The listing builds one solid part. Answer for the finished solid, in the listing's coordinates (mm). Face numbers are marked on the shaded views. A direction names the side the tool comes from. Coordinates: 2 decimals unless noted, no trailing zeros. Loops run counter-clockwise (first coordinate to the right, second up) from the corner with the lowest first, then second, coordinate; pieces in that order, holes last. Notation, with made-up numbers: M 67,-18.5 L 115,-18.5 A27 ccw 115,16.5 Z; hole C 89,59 d3. An arc over 180 degrees is marked long. Return JSON: item names as keys, results as strings. Group by question number.
1. The mould has two halves that part along X. Classify the marked faces 1, 2 and 3: pulls with the +X half, pulls with the -X half, needs draft (parallel to the pull), parting line crosses it, or undercut.
2. Section D-D (y = 25.5) is taken. Write down the section's boundary in (x, z), then the cut area to 3 significant figures.
3. Which of the six approach directions +Z, -Z, +X, -X, +Y, -Y give full straight-line access (tool end or side, diameter ignored) to the marked faces 4, 5 and 6?
4. Given P1, Ø1.5, axis at x = 61.5, z = 3.5, coming from the -Y side; P2, Ø24, axis at x = 61.5, z = -19, coming from the +Y side; P3, Ø5, axis at y = 55, z = -24, coming from the -X side; P4, Ø20, axis at x = 118.5, z = 8.5, coming from the +Y side, each flat-ended and moving along its own axis, determine where each tip first touches the part or whether it passes through.
5. Straight lines are drawn through the part: L1, parallel to X at y = 23, z = 0; L2, parallel to Z at x = 34, y = 43; L3, parallel to X at y = 43, z = 0. For each, find the intervals that lie inside material, in ascending order. Write a range as from..to.
6. Section A-A (x = 70) is taken. Write down the section's boundary in (y, z).
7. Section C-C (z = 0) is taken. Write down the section's boundary in (x, y), then the cut area to 3 significant figures.
8. Section B-B (y = 47) is taken. Write down the section's boundary in (x, z), then the cut area to 3 significant figures.
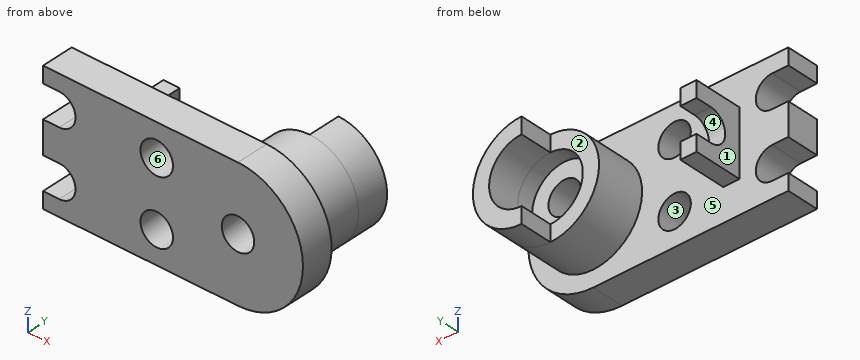
```python
from build123d import *

# Parameters (mm, degrees)
BOSS_EXTRUDE1_DEPTH = 20
CUT_EXTRUDE1_DEPTH  = 20
SKETCH4_R           = 10
CUT_EXTRUDE2_DEPTH  = 20
SKETCH5_R           = 20
BOSS_EXTRUDE2_DEPTH = 20
SKETCH6_R           = 30
BOSS_EXTRUDE3_DEPTH = 30
SKETCH7_R           = 20
CUT_EXTRUDE3_DEPTH  = 10
SKETCH8_R           = 10
CUT_EXTRUDE4_DEPTH  = 72
BOSS_EXTRUDE4_DEPTH = 20
SKETCH10_W          = 10
SKETCH10_H          = 40
BOSS_EXTRUDE5_DEPTH = 30
CUT_EXTRUDE5_DEPTH  = 30


with BuildPart() as part:
    # Sketch2 → Boss-Extrude1 (new body)
    with BuildSketch(Plane(origin=(0, 0, 0), x_dir=(1, 0, 0), z_dir=(0, 1, 0))):
        with BuildLine():
            Line((0, 40), (0, -40))
            Line((0, -40), (120, -40))
            ThreePointArc((120, -40), (160, 0), (120, 40))
            Line((120, 40), (0, 40))
        make_face()
    extrude(amount=BOSS_EXTRUDE1_DEPTH)

    # Sketch3 → Cut-Extrude1 (cut)
    with BuildSketch(Plane(origin=(0, 20, 0), x_dir=(1, 0, 0), z_dir=(0, 1, 0))):
        with BuildLine():
            Line((0, 30), (10, 30))
            ThreePointArc((10, 30), (20, 20), (10, 10))
            Line((10, 10), (0, 10))
            Line((0, 10), (0, 30))
        make_face()
        with BuildLine():
            Line((0, -10), (10, -10))
            ThreePointArc((10, -10), (20, -20), (10, -30))
            Line((10, -30), (0, -30))
            Line((0, -30), (0, -10))
        make_face()
    extrude(amount=-CUT_EXTRUDE1_DEPTH, mode=Mode.SUBTRACT)

    # Sketch4 → Cut-Extrude2 (cut)
    with BuildSketch(Plane(origin=(0, 20, 0), x_dir=(1, 0, 0), z_dir=(0, 1, 0))):
        with Locations(Location((70, 20, 0), (0, 0, 270))):
            Circle(SKETCH4_R)
        with Locations(Location((70, -20, 0), (0, 0, 270))):
            Circle(SKETCH4_R)
    extrude(amount=-CUT_EXTRUDE2_DEPTH, mode=Mode.SUBTRACT)

    # Sketch5 → Boss-Extrude2 (add)
    with BuildSketch(Plane(origin=(0, 20, 0), x_dir=(1, 0, 0), z_dir=(0, 1, 0))):
        with Locations(Location((120, 0, 0), (0, 0, 90))):
            Circle(SKETCH5_R)
    extrude(amount=BOSS_EXTRUDE2_DEPTH)

    # Sketch6 → Boss-Extrude3 (add)
    with BuildSketch(Plane(origin=(0, 20, 0), x_dir=(1, 0, 0), z_dir=(0, 1, 0))):
        with Locations(Location((120, 0, 0), (0, 0, 90))):
            Circle(SKETCH6_R)
    extrude(amount=BOSS_EXTRUDE3_DEPTH)

    # Sketch7 → Cut-Extrude3 (cut)
    with BuildSketch(Plane(origin=(0, 50, 0), x_dir=(1, 0, 0), z_dir=(0, 1, 0))):
        with Locations(Location((120, 0, 0), (0, 0, 270))):
            Circle(SKETCH7_R)
    extrude(amount=-CUT_EXTRUDE3_DEPTH, mode=Mode.SUBTRACT)

    # Sketch8 → Cut-Extrude4 (cut)
    with BuildSketch(Plane(origin=(0, 40, 0), x_dir=(1, 0, 0), z_dir=(0, 1, 0))):
        with Locations(Location((120, 0, 0), (0, 0, 270))):
            Circle(SKETCH8_R)
    extrude(amount=-CUT_EXTRUDE4_DEPTH, mode=Mode.SUBTRACT)

    # Sketch9 → Boss-Extrude4 (add)
    with BuildSketch(Plane(origin=(0, 50, 0), x_dir=(1, 0, 0), z_dir=(0, 1, 0))):
        with BuildLine():
            Line((120, 20), (120, 30))
            ThreePointArc((120, 30), (150, 0), (120, -30))
            Line((120, -30), (120, -20))
            ThreePointArc((120, -20), (140, 0), (120, 20))
        make_face()
    extrude(amount=BOSS_EXTRUDE4_DEPTH)

    # Sketch10 → Boss-Extrude5 (add)
    with BuildSketch(Plane(origin=(0, 20, 0), x_dir=(1, 0, 0), z_dir=(0, 1, 0))):
        with Locations((35, 0)):
            Rectangle(SKETCH10_W, SKETCH10_H)
    extrude(amount=BOSS_EXTRUDE5_DEPTH)

    # Sketch11 → Cut-Extrude5 (cut)
    with BuildSketch(Plane.ZY.offset(-30)):
        with BuildLine():
            Line((-10, 50), (-10, 40))
            ThreePointArc((-10, 40), (0, 30), (10, 40))
            Line((10, 40), (10, 50))
            Line((10, 50), (-10, 50))
        make_face()
    extrude(amount=-CUT_EXTRUDE5_DEPTH, mode=Mode.SUBTRACT)


solid = part.part
```
Worked out:
{
 "1": {"face 1": "pulls with the -X half", "face 2": "needs draft", "face 3": "undercut"},
 "2": {"outline": "M 30,-20 L 40,-20 L 40,20 L 30,20 Z; C 120,0 d60; hole C 120,0 d20", "area": "2,910 mm^2"},
 "3": {"face 4": "-X, +Y", "face 5": "+Y", "face 6": "+Y, -Y"},
 "4": {"P1": "y = 0", "P2": "y = 20", "P3": "x = 120", "P4": "y = 40"},
 "5": {"L1": "30..40, 90..110, 130..150", "L2": "-20..-10, 10..20", "L3": "90..100, 140..150"},
 "6": {"outline": "M 0,-40 L 20,-40 L 20,-30 L 0,-30 Z; M 0,-10 L 20,-10 L 20,10 L 0,10 Z; M 0,30 L 20,30 L 20,40 L 0,40 Z"},
 "7": {"outline": "M 0,0 L 110,0 L 110,40 L 100,40 L 100,50 L 90,50 L 90,20 L 40,20 L 40,30 L 30,30 L 30,20 L 0,20 Z; M 130,0 L 160,0 L 160,20 L 150,20 L 150,70 L 140,70 L 140,40 L 130,40 Z", "area": "4,100 mm^2"},
 "8": {"outline": "M 30,-20 L 40,-20 L 40,-10 L 30,-10 Z; M 30,10 L 40,10 L 40,20 L 30,20 Z; C 120,0 d60; hole C 120,0 d40", "area": "1,770 mm^2"}
}
